Model file for the job. Use its own axes, mm. A direction names the side the tool comes from. Coordinates: 2 decimals unless noted, no trailing zeros. Loops run counter-clockwise (first coordinate to the right, second up) from the corner with the lowest first, then second, coordinate; pieces in that order, holes last. Notation, with made-up numbers: (-1, 74) -> (39, 74) arc R11 cw to (39, 88) -> close; hole circle Ø10 at (5, 87). An arc over 180 degrees is marked (long way). Use one line per item in the form item = value.
```python
from build123d import *

# Parameters (mm, degrees)
SKETCH1_R           = 12
SKETCH1_R_2         = 1.5
SKETCH1_R_3         = 4.25
BOSS_EXTRUDE1_DEPTH = 2.6
SKETCH2_R           = 1.75
BOSS_EXTRUDE2_DEPTH = 4.4
BOSS_EXTRUDE3_DEPTH = 2.6
BOSS_EXTRUDE4_START = 10
SKETCH5_R           = 2.001113277
BOSS_EXTRUDE4_DEPTH = 10
SKETCH6_R           = 5
BOSS_EXTRUDE5_DEPTH = 2
FILLET1_R           = 5


with BuildPart() as part:
    # Sketch1 → Boss-Extrude1 (new body)
    with BuildSketch(Plane(origin=(0, 0, 0), x_dir=(1, 0, 0), z_dir=(0, 1, 0))):
        with Locations(Location((0, 0, 0), (0, 0, 270))):
            Circle(SKETCH1_R)
        with Locations(Location((0, 8, 0), (0, 0, 270))):
            Circle(SKETCH1_R_2, mode=Mode.SUBTRACT)
        with Locations(Location((9.5, 0, 0), (0, 0, 270))):
            Circle(SKETCH1_R_2, mode=Mode.SUBTRACT)
        with Locations(Location((0, -8, 0), (0, 0, 270))):
            Circle(SKETCH1_R_2, mode=Mode.SUBTRACT)
        with Locations(Location((-9.5, 0, 0), (0, 0, 270))):
            Circle(SKETCH1_R_2, mode=Mode.SUBTRACT)
        with Locations(Location((0, 0, 0), (0, 0, 270))):
            Circle(SKETCH1_R_3, mode=Mode.SUBTRACT)
    extrude(amount=BOSS_EXTRUDE1_DEPTH)

    # Sketch2 → Boss-Extrude2 (add)
    with BuildSketch(Plane(origin=(0, 2.6, 0), x_dir=(1, 0, 0), z_dir=(0, 1, 0))):
        with Locations(Location((-7.071067812, 7.071067812, 0), (0, 0, 270))):
            Circle(SKETCH2_R)
        with Locations(Location((7.071067812, 7.071067812, 0), (0, 0, 270))):
            Circle(SKETCH2_R)
        with Locations(Location((7.071067812, -7.071067812, 0), (0, 0, 270))):
            Circle(SKETCH2_R)
        with Locations(Location((-7.071067812, -7.071067812, 0), (0, 0, 270))):
            Circle(SKETCH2_R)
    extrude(amount=BOSS_EXTRUDE2_DEPTH)

    # Sketch3 → Boss-Extrude3 (add)
    with BuildSketch(Plane(origin=(0, 2.6, 0), x_dir=(1, 0, 0), z_dir=(0, 1, 0))):
        with BuildLine():
            Line((-22.580224051, 19.751796926), (-9.780813828, 6.952386703))
            ThreePointArc((-9.780813828, 6.952386703), (-8.455336604, 8.455336604), (-6.952386703, 9.780813828))
            Line((-6.952386703, 9.780813828), (-19.751796926, 22.580224051))
            ThreePointArc((-19.751796926, 22.580224051), (-22.628204204, 22.628204204), (-22.580224051, 19.751796926))
        make_face()
        with BuildLine():
            Line((19.751796926, 22.580224051), (6.952386703, 9.780813828))
            ThreePointArc((6.952386703, 9.780813828), (8.455336604, 8.455336604), (9.780813828, 6.952386703))
            Line((9.780813828, 6.952386703), (22.580224051, 19.751796926))
            ThreePointArc((22.580224051, 19.751796926), (22.628204204, 22.628204204), (19.751796926, 22.580224051))
        make_face()
        with BuildLine():
            Line((22.580224051, -19.751796926), (9.780813828, -6.952386703))
            ThreePointArc((9.780813828, -6.952386703), (8.455336604, -8.455336604), (6.952386703, -9.780813828))
            Line((6.952386703, -9.780813828), (19.751796926, -22.580224051))
            ThreePointArc((19.751796926, -22.580224051), (22.628204204, -22.628204204), (22.580224051, -19.751796926))
        make_face()
        with BuildLine():
            Line((-19.751796926, -22.580224051), (-6.952386703, -9.780813828))
            ThreePointArc((-6.952386703, -9.780813828), (-8.455336604, -8.455336604), (-9.780813828, -6.952386703))
            Line((-9.780813828, -6.952386703), (-22.580224051, -19.751796926))
            ThreePointArc((-22.580224051, -19.751796926), (-22.628204204, -22.628204204), (-19.751796926, -22.580224051))
        make_face()
    extrude(amount=-BOSS_EXTRUDE3_DEPTH)

    # Sketch5 → Boss-Extrude4 (add)
    with BuildSketch(Plane(origin=(0, 2.6, 0), x_dir=(1, 0, 0), z_dir=(0, 1, 0)).offset(BOSS_EXTRUDE4_START)):
        with Locations(Location((-21.213203436, 21.213203436, 0), (0, 0, 270))):
            Circle(SKETCH5_R)
        with Locations(Location((21.213203436, 21.213203436, 0), (0, 0, 270))):
            Circle(SKETCH5_R)
        with Locations(Location((21.213203436, -21.213203436, 0), (0, 0, 270))):
            Circle(SKETCH5_R)
        with Locations(Location((-21.213203436, -21.213203436, 0), (0, 0, 270))):
            Circle(SKETCH5_R)
    extrude(amount=-BOSS_EXTRUDE4_DEPTH)

    # Sketch6 → Boss-Extrude5 (add)
    with BuildSketch(Plane(origin=(0, 12.6, 0), x_dir=(1, 0, 0), z_dir=(0, 1, 0))):
        with Locations(Location((21.213203436, -21.213203436, 0), (0, 0, 270))):
            Circle(SKETCH6_R)
        with Locations(Location((21.213203436, 21.213203436, 0), (0, 0, 270))):
            Circle(SKETCH6_R)
        with Locations(Location((-21.213203436, 21.213203436, 0), (0, 0, 270))):
            Circle(SKETCH6_R)
        with Locations(Location((-21.213203436, -21.213203436, 0), (0, 0, 270))):
            Circle(SKETCH6_R)
    extrude(amount=-BOSS_EXTRUDE5_DEPTH)

    # Fillet1
    fillet1_edges = [part.edges().sort_by_distance(p)[0] for p in [
        (-6.952386703, 1.3, -9.780813828),
        (-9.780813828, 1.3, -6.952386703),
        (9.780813828, 1.3, -6.952386703),
        (6.952386703, 1.3, -9.780813828),
        (6.952386703, 1.3, 9.780813828),
        (9.780813828, 1.3, 6.952386703),
        (-9.780813828, 1.3, 6.952386703),
        (-6.952386703, 1.3, 9.780813828),
    ]]
    fillet(fillet1_edges, radius=FILLET1_R)

    # Fillet2: read off the stored shape, not the designer's step
    # Fillet2 outline → Fillet2 (revolve)
    with BuildSketch(Plane(origin=(-21.213203436, 0, 21.213203436), x_dir=(1, 0, 0), z_dir=(0, 0, 1))):
        with BuildLine():
            ThreePointArc((2.001113277, 6.01791034), (2.817480503, 8.756014941), (5, 10.6))
            Line((5, 10.6), (2.001113277, 10.6))
            Line((2.001113277, 10.6), (2.001113277, 6.01791034))
        make_face()
    revolve(axis=Axis((-21.213203436, 0, 21.213203436), (0, 1, 0)))

    # Fillet2 2 outline → Fillet2 2 (revolve)
    with BuildSketch(Plane(origin=(21.213203436, 0, 21.213203436), x_dir=(1, 0, 0), z_dir=(0, 0, 1))):
        with BuildLine():
            ThreePointArc((2.001113277, 6.01791034), (2.817480503, 8.756014941), (5, 10.6))
            Line((5, 10.6), (2.001113277, 10.6))
            Line((2.001113277, 10.6), (2.001113277, 6.01791034))
        make_face()
    revolve(axis=Axis((21.213203436, 0, 21.213203436), (0, 1, 0)))

    # Fillet2 3 outline → Fillet2 3 (revolve)
    with BuildSketch(Plane(origin=(21.213203436, 0, -21.213203436), x_dir=(1, 0, 0), z_dir=(0, 0, 1))):
        with BuildLine():
            ThreePointArc((2.001113277, 6.01791034), (2.817480503, 8.756014941), (5, 10.6))
            Line((5, 10.6), (2.001113277, 10.6))
            Line((2.001113277, 10.6), (2.001113277, 6.01791034))
        make_face()
    revolve(axis=Axis((21.213203436, 0, -21.213203436), (0, 1, 0)))

    # Fillet2 4 outline → Fillet2 4 (revolve)
    with BuildSketch(Plane(origin=(-21.213203436, 0, -21.213203436), x_dir=(1, 0, 0), z_dir=(0, 0, 1))):
        with BuildLine():
            ThreePointArc((2.001113277, 6.01791034), (2.817480503, 8.756014941), (5, 10.6))
            Line((5, 10.6), (2.001113277, 10.6))
            Line((2.001113277, 10.6), (2.001113277, 6.01791034))
        make_face()
    revolve(axis=Axis((-21.213203436, 0, -21.213203436), (0, 1, 0)))


solid = part.part
```
Q1. Which spindle directions (+Z, -Z, +X, -X, +Y, -Y) get a long thin tool onto all of the face, cutting with end or side? Do faces 4 (the face through (-14.72, 1.32, 17.55)), 5 (the face through (-17.4, 1.32, 14.57)), 6 (the face through (17.55, 1.32, 14.72)), 7 (the face through (8, 1, 0)), 8 (the face through (-8.62, 4.77, -6.26)). Say none if no direction does.
Result:
face_4 = +Z, -Y
face_5 = -X, -Y
face_6 = +X, -Y
face_7 = +Y, -Y
face_8 = +Y
Q2. Band-saw the part on C-C, the plane y = 4.75. Write the cut outline in (x, z), and give its area (3 significant figures).
Result:
outline = circle Ø4 at (-21.21, -21.21); circle Ø4 at (-21.21, 21.21); circle Ø3.5 at (-7.07, -7.07); circle Ø3.5 at (-7.07, 7.07); circle Ø3.5 at (7.07, -7.07); circle Ø3.5 at (7.07, 7.07); circle Ø4 at (21.21, -21.21); circle Ø4 at (21.21, 21.21)
area = 88.8 mm2
Q3. Band-saw the part on B-B, the plane x = 0. Write the cut outline in (y, z).
Result:
outline = (0, -12) -> (2.6, -12) -> (2.6, -9.5) -> (0, -9.5) -> close; (0, -6.5) -> (2.6, -6.5) -> (2.6, -4.25) -> (0, -4.25) -> close; (0, 4.25) -> (2.6, 4.25) -> (2.6, 6.5) -> (0, 6.5) -> close; (0, 9.5) -> (2.6, 9.5) -> (2.6, 12) -> (0, 12) -> close
Q4. Band-saw the part on A-A, the plane z = 0. Write the cut outline in (x, y).
Result:
outline = (-12, 0) -> (-11, 0) -> (-11, 2.6) -> (-12, 2.6) -> close; (-8, 0) -> (-4.25, 0) -> (-4.25, 2.6) -> (-8, 2.6) -> close; (4.25, 0) -> (8, 0) -> (8, 2.6) -> (4.25, 2.6) -> close; (11, 0) -> (12, 0) -> (12, 2.6) -> (11, 2.6) -> close
Q5. Wall check: line 1 along X through (y, z) = (0.7, 0); line 2 along Y through (x, z) = (-9.5, -9); line 3 along Z through (x, y) = (-22.5, 5.5). Give the ranges that are in metal, low to high.
Result:
line_1 = -12 to -11, -8 to -4.25, 4.25 to 8, 11 to 12
line_2 = 0 to 2.6
line_3 = -22.75 to -19.68, 19.68 to 22.75
Q6. Mould opens along Z. For faces 1 (the face through (-20.99, 11.61, 16.22)), 2 (the face through (0, 1, 12)), 3 (the face through (7, 7, 7)) say: released by +Z, released by -Z, zero draft, split by the parting line, or undercut.
Result:
face_1 = undercut
face_2 = released by +Z
face_3 = zero draft
Q7. Band-saw the part on D-D, the plane z = 13.5. Write the cut outline in (x, y).
Result:
outline = (-16.33, 0) -> (-10.67, 0) -> (-10.67, 2.6) -> (-16.33, 2.6) -> close; (10.67, 0) -> (16.33, 0) -> (16.33, 2.6) -> (10.67, 2.6) -> close
Q8. Pin check, flat tips, straight feed: pin 1 Ø1.8 at (x, z) = (9.5, 0) entering from +Y; pin 2 Ø4 at (y, z) = (4.5, 3.5) entering from -X; pin 3 Ø3 at (x, z) = (7, 7.5) entering from +Y; pin 4 Ø3.5 at (x, z) = (0, -8) entering from +Y. Stop position of each tip, or through.
Result:
pin_1 = through
pin_2 = -11.65
pin_3 = 7
pin_4 = 2.6
